```python
from build123d import *

# Parameters (mm, degrees)
SKETCH1_W           = 80
SKETCH1_H           = 70
BOSS_EXTRUDE1_DEPTH = 4
SKETCH1_3_W         = 4
SKETCH1_3_H         = 70
BOSS_EXTRUDE2_DEPTH = 80
SKETCH1_4_W         = 4
SKETCH1_4_H         = 70
BOSS_EXTRUDE3_DEPTH = 25
SKETCH2_R           = 4
CUT_EXTRUDE1_DEPTH  = 134.041346957
SKETCH3_R           = 3.25
CUT_EXTRUDE2_DEPTH  = 131.675169791
SKETCH3_3_R         = 14.2875
SKETCH3_3_R_2       = 3.25
CUT_EXTRUDE3_DEPTH  = 1
SKETCH1_5_W         = 25.2
SKETCH1_5_H         = 70
BOSS_EXTRUDE4_DEPTH = 6.84


with BuildPart() as part:
    # Sketch1 → Boss-Extrude1 (new body)
    with BuildSketch(Plane(origin=(0, 0, 0), x_dir=(1, 0, 0), z_dir=(0, 1, 0))):
        with Locations((40, 35)):
            Rectangle(SKETCH1_W, SKETCH1_H)
    extrude(amount=BOSS_EXTRUDE1_DEPTH)

    # Sketch1_3 → Boss-Extrude2 (add)
    with BuildSketch(Plane(origin=(0, 0, 0), x_dir=(1, 0, 0), z_dir=(0, 1, 0))):
        with Locations((2, 35)):
            Rectangle(SKETCH1_3_W, SKETCH1_3_H)
    extrude(amount=BOSS_EXTRUDE2_DEPTH)

    # Sketch1_4 → Boss-Extrude3 (add)
    with BuildSketch(Plane(origin=(0, 0, 0), x_dir=(1, 0, 0), z_dir=(0, 1, 0))):
        with Locations((78, 35)):
            Rectangle(SKETCH1_4_W, SKETCH1_4_H)
        with Locations((48.8, 35)):
            Rectangle(SKETCH1_4_W, SKETCH1_4_H)
    extrude(amount=-BOSS_EXTRUDE3_DEPTH)

    # Sketch2 → Cut-Extrude1 (cut, through all)
    with BuildSketch(Plane(origin=(80, 0, 0), x_dir=(0, 0, -1), z_dir=(1, 0, 0))):
        with Locations(Location((9.8, -12, 0), (0, 0, 180))):
            Circle(SKETCH2_R)
        with Locations(Location((60.2, -12, 0), (0, 0, 180))):
            Circle(SKETCH2_R)
    extrude(amount=-CUT_EXTRUDE1_DEPTH, mode=Mode.SUBTRACT)

    # Sketch3 → Cut-Extrude2 (cut, through all)
    with BuildSketch(Plane(origin=(4, 0, 0), x_dir=(0, 0, -1), z_dir=(1, 0, 0))):
        with Locations((35, 37.756)):
            Circle(SKETCH3_R)
    extrude(amount=-CUT_EXTRUDE2_DEPTH, mode=Mode.SUBTRACT)

    # Sketch3_3 → Cut-Extrude3 (cut)
    with BuildSketch(Plane(origin=(4, 0, 0), x_dir=(0, 0, -1), z_dir=(1, 0, 0))):
        with Locations((35, 29.4)):
            Circle(SKETCH3_3_R)
        with Locations((35, 37.756)):
            Circle(SKETCH3_3_R_2, mode=Mode.SUBTRACT)
    extrude(amount=-CUT_EXTRUDE3_DEPTH, mode=Mode.SUBTRACT)

    # Sketch1_5 → Boss-Extrude4 (add)
    with BuildSketch(Plane(origin=(0, 0, 0), x_dir=(1, 0, 0), z_dir=(0, 1, 0))):
        with Locations((63.4, 35)):
            Rectangle(SKETCH1_5_W, SKETCH1_5_H)
    extrude(amount=-BOSS_EXTRUDE4_DEPTH)


solid = part.part
```
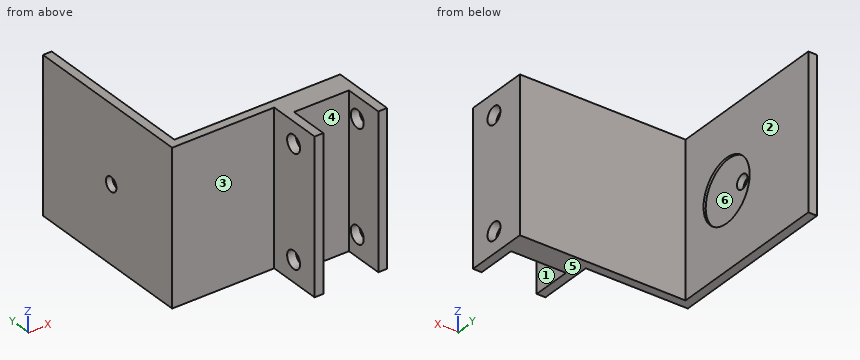
CAD build for the part. Positions are in the model's coordinates, mm. Face numbers are marked on the shaded views. A direction names the side the tool comes from. Give positions to 0.01 mm unless a question says otherwise; leave off trailing zeros. Order: outer loops, then holes, each group sorted by start corner. A loop starts at its lowest first (then second) coordinate and runs counter-clockwise, first axis right, second up.
(1) Tool access for the marked faces 1, 2 and 3: list every direction of +Z, -Z, +X, -X, +Y, -Y with a clear straight run to the whole face (end or side of a thin tool).
(2) Drill centre lines: L1, parallel to Z at x = 78.1, y = -12; L2, parallel to Y at x = 79, z = -9.8; L3, parallel to X at y = -17, z = -21.5. Where is each one in solid material? Low to high.
(3) Mould opens along X. For the marked faces 4, 5 and 6 say: released by +X, released by -X, zero draft, split by the parting line, or undercut.
(4) Saw through at A-A, the plane z = -35. Give the cut face in (x, y).
(5) Flat gauge pins, fed straight in: pin 1 (21 mm diameter, centred on y = 25, z = -34, fed in from +X); pin 2 (6 mm diameter, centred on x = 58, z = -43.5, fed in from +Y); pin 3 (8.5 mm diameter, centred on y = 23.5, z = -34.5, fed in from +X); pin 4 (7 mm diameter, centred on y = -12, z = -9.8, fed in from -X). Where does each tip first touch, or does it go through?
(6) Saw through at D-D, the plane x = 9. Give the cut face in (y, z), then the cut area to 3 significant figures.
(7) Saw through at C-C, the plane y = 29.4. Give the cut face in (x, z).
(8) Saw through at B-B, the plane z = -9.8. Give the cut face in (x, y), then the cut area to 3 significant figures.
Results found:
1. face 1: +Z, -Z, -Y
1. face 2: +Z, -Z, +X, +Y
1. face 3: +Z, -Z, -X, -Y
2. L1: z = -70 to -64.2, -56.2 to -13.8, -5.8 to 0
2. L2: y = -25 to -16, -8 to 4
2. L3: x = 46.8 to 50.8, 76 to 80
3. face 4: undercut
3. face 5: zero draft
3. face 6: released by +X
4. outline: (0, 0) - (46.8, 0) - (46.8, -25) - (50.8, -25) - (50.8, -6.84) - (76, -6.84) - (76, -25) - (80, -25) - (80, 4) - (4, 4) - (4, 15.11) - (3, 15.11) - (3, 34.51) - (0, 34.51) - close; (0, 41.01) - (3, 41.01) - (3, 43.69) - (4, 43.69) - (4, 80) - (0, 80) - close
5. pin 1: stops at x = 4
5. pin 2: stops at y = 4
5. pin 3: stops at x = 3
5. pin 4: passes through
6. outline: (0, -70) - (4, -70) - (4, 0) - (0, 0) - close
6. area: 280 mm2
7. outline: (0, -70) - (4, -70) - (4, -49.29) - (3, -49.29) - (3, -20.71) - (4, -20.71) - (4, 0) - (0, 0) - close
8. outline: (0, 0) - (46.8, 0) - (46.8, -8) - (50.8, -8) - (50.8, -6.84) - (76, -6.84) - (76, -8) - (80, -8) - (80, 4) - (4, 4) - (4, 80) - (0, 80) - close; (46.8, -25) - (50.8, -25) - (50.8, -16) - (46.8, -16) - close; (76, -25) - (80, -25) - (80, -16) - (76, -16) - close
8. area: 932 mm2
